```python
from build123d import *

# Parameters (mm, degrees)
F0_W     = 25
F0_H     = 25
F0_R     = 3
F0_R_2   = 2.943766
F1_DEPTH = 25


with BuildPart() as f1:
    # F0 (on Right) → F1 (new body)
    with BuildSketch(Plane.YZ):
        Polygon((28.680211, 1900.875823), (3.680211, 1908.51909), (3.680211, -277.290163), (28.680211, -277.290163), align=None)
        Polygon((160.387475, 2140.847163), (3.680211, 1908.51909), (28.680211, 1900.875823), (173.680211, 2115.847163), align=None)
        Polygon((296.972947, 2140.847163), (160.387475, 2140.847163), (173.680211, 2115.847163), (283.680211, 2115.847163), align=None)
        Polygon((453.680211, 1908.51909), (296.972947, 2140.847163), (283.680211, 2115.847163), (428.680211, 1900.875823), align=None)
        Polygon((453.680211, 1821.632886), (453.680211, 1908.51909), (428.680211, 1900.875823), (428.680211, 1821.632886), align=None)
        with Locations((441.180211, 1809.132886)):
            Rectangle(F0_W, F0_H)
        with BuildLine():
            Line((476.079169, 1779.894328), (481.180211, 1796.632886))
            Line((481.180211, 1796.632886), (474.974158, 1781.067371))
            Line((474.974158, 1781.067371), (448.744883, 1781.067371))
            ThreePointArc((448.744883, 1781.067371), (448.772956, 1780.831839), (448.782334, 1780.594826))
            ThreePointArc((448.782334, 1780.594826), (445.54532, 1777.604203), (442.819784, 1781.067371))
            Line((442.819784, 1781.067371), (412.465903, 1781.067371))
            Line((412.465903, 1781.067371), (401.180211, 1796.632886))
            Line((401.180211, 1796.632886), (410.844222, 1779.894328))
            Line((410.844222, 1779.894328), (364.232844, 1699.161054))
            Line((364.232844, 1699.161054), (341.180211, 1692.709837))
            Line((341.180211, 1692.709837), (541.180211, 1692.709837))
            Line((541.180211, 1692.709837), (522.690546, 1699.161054))
            Line((522.690546, 1699.161054), (476.079169, 1779.894328))
        make_face()
        with Locations((489.227206, 1706.84576)):
            Circle(F0_R, mode=Mode.SUBTRACT)
        with Locations((468.309313, 1741.440773)):
            Circle(F0_R, mode=Mode.SUBTRACT)
        Polygon((541.180211, 1692.709837), (481.180211, 1796.632886), (476.079169, 1779.894328), (522.690546, 1699.161054), align=None)
        with BuildLine():
            Line((481.180211, 1796.632886), (453.680211, 1796.632886))
            Line((453.680211, 1796.632886), (428.680211, 1796.632886))
            Line((428.680211, 1796.632886), (401.180211, 1796.632886))
            Line((401.180211, 1796.632886), (412.465903, 1781.067371))
            Line((412.465903, 1781.067371), (442.819784, 1781.067371))
            ThreePointArc((442.819784, 1781.067371), (445.782334, 1783.594826), (448.744883, 1781.067371))
            Line((448.744883, 1781.067371), (474.974158, 1781.067371))
            Line((474.974158, 1781.067371), (481.180211, 1796.632886))
        make_face()
        with Locations((467.166099, 1789.444685)):
            Circle(F0_R_2, mode=Mode.SUBTRACT)
        Polygon((410.844222, 1779.894328), (401.180211, 1796.632886), (341.180211, 1692.709837), (364.232844, 1699.161054), align=None)
    extrude(amount=F1_DEPTH)


solid = f1.part
```
Can you work these out from the model? Positions are in its coordinate system, mm. A direction names the side the tool comes from. Coordinates: 2 decimals unless noted, no trailing zeros. Loops run counter-clockwise (first coordinate to the right, second up) from the corner with the lowest first, then second, coordinate; pieces in that order, holes last.
1) For pin 1 (12.5 mm diameter, centred on x = 8.5, z = 1864, fed in from +Y); pin 2 (9.5 mm diameter, centred on y = 489.23, z = 1706.85, fed in from +X); pin 3 (8 mm diameter, centred on x = 13, z = 1107, fed in from +Y); pin 4 (3 mm diameter, centred on x = 5, y = 208.5, fed in from -Z), each with a flat end and sliding along its axis, tell me the tip position at first contact or that it passes through.
2) I need wall thicknesses on probe 1 along Y at (x, z) = (16, -174.5); probe 2 along Z at (x, y) = (7, 203.5); probe 3 along Y at (x, z) = (6.75, 1911). Which ranges of each line are inside material? Lowest first, please.
3) Imagine slicing it at C-C on z = 1342.5. List the corners of the cut face in (x, y) for me, plus the area to 3 significant figures.
4) Thinking about a two-plate mould opening in Y: for faces 1 (the flat face through (25, 12, 1206)), 2 (the flat face through (12.3, 371.6, 1745.4)), 3 (the flat face through (12.32, 83.13, 2026.31)), which applies, pulls with the +Y half, pulls with the -Y half, needs draft (parallel to the pull), parting line crosses it, or undercut?
5) Imagine slicing it at A-A on x = 16. List the corners of the cut face in (y, z) for me.
6) Imagine slicing it at B-B on y = 238. List the corners of the cut face in (x, z) for me.
7) Which directions (+Z, -Z, +X, -X, +Y, -Y) give clear straight access to the entire face, cutting with the end or side of a thin tool? Please do faces 4 (the flat face through (12.325, 511.6, 1743.944)), 5 (the flat face through (12.325, 355.165, 2009.866)), 6 (the flat face through (12.325, 100.165, 2006.857)).
Completed:
1. pin 1: stops at y = 453.68
1. pin 2: stops at x = 25
1. pin 3: stops at y = 28.68
1. pin 4: stops at z = 2115.85
2. probe 1: y = 3.68 to 28.68
2. probe 2: z = 2115.85 to 2140.85
2. probe 3: y = 5.35 to 35.51, 421.85 to 452.01
3. outline: (0, 3.68) - (25, 3.68) - (25, 28.68) - (0, 28.68) - close
3. area: 625 mm2
4. face 1: needs draft
4. face 2: undercut
4. face 3: pulls with the -Y half
5. outline: (3.68, -277.29) - (28.68, -277.29) - (28.68, 1900.88) - (173.68, 2115.85) - (283.68, 2115.85) - (428.68, 1900.88) - (428.68, 1796.63) - (401.18, 1796.63) - (341.18, 1692.71) - (541.18, 1692.71) - (481.18, 1796.63) - (453.68, 1796.63) - (453.68, 1908.52) - (296.97, 2140.85) - (160.39, 2140.85) - (3.68, 1908.52) - close; hole (448.74, 1781.07) arc R3 ccw (long way) to (448.78, 1780.59) arc R3 ccw to start; hole circle Ø5.89 at (467.17, 1789.44); hole circle Ø6 at (468.31, 1741.44); hole circle Ø6 at (489.23, 1706.85)
6. outline: (0, 2115.85) - (25, 2115.85) - (25, 2140.85) - (0, 2140.85) - close
7. face 4: +Z, +X, -X, +Y
7. face 5: +X, -X
7. face 6: -Z, +X, -X
